Autodesk Inventor part; units mm, degrees
ref_plane "YZ Plane" through (0, 0, 0) normal (1, 0, 0) x (0, 1, 0)
ref_plane "XZ Plane" through (0, 0, 0) normal (0, 1, 0) x (-1, 0, 0)
ref_plane "XY Plane" through (0, 0, 0) normal (0, 0, 1) x (1, 0, 0)
sketch "Sketch1" plane through (0, 0, 0) normal (0, 1, 0) x (-1, 0, 0)
  arc A0 (1.4918, 12.1563) -> (-1.4918, 12.1563) centre (0, 12) ccw
  arc A1 (-1.4918, -12.1563) -> (1.4918, -12.1563) centre (0, -12) ccw
  line L0 (0, -12) -> (0, 12) construction
  line L1 (-2.735, 0.2865) -> (-1.4918, 12.1563)
  line L2 (1.4918, -12.1563) -> (2.735, -0.2865)
  line L3 (-1.4918, -12.1563) -> (-2.735, -0.2865)
  line L4 (2.735, 0.2865) -> (1.4918, 12.1563)
  arc A2 (-2.735, 0.2865) -> (-2.735, -0.2865) centre (0, 0) ccw
  arc A3 (2.735, -0.2865) -> (2.735, 0.2865) centre (0, 0) ccw
  line L5 (2.75, 0) -> (-2.75, 0) construction
  line L6 (-3.0334, -0.3177) -> (-1.7902, -12.1875)
  arc A4 (-1.7902, -12.1875) -> (1.7902, -12.1875) centre (0, -12) ccw
  line L7 (1.7902, -12.1875) -> (3.0334, -0.3177)
  arc A5 (3.0334, -0.3177) -> (3.0334, 0.3177) centre (0, 0) ccw
  line L8 (3.0334, 0.3177) -> (1.7902, 12.1875)
  arc A6 (1.7902, 12.1875) -> (-1.7902, 12.1875) centre (0, 12) ccw
  line L9 (-1.7902, 12.1875) -> (-3.0334, 0.3177)
  arc A7 (-3.0334, 0.3177) -> (-3.0334, -0.3177) centre (0, 0) ccw
  line L10 (-4.25, 27.45) -> (4.25, 27.45)
  line L11 (4.25, 27.45) -> (4.25, 48.45)
  line L12 (4.25, 48.45) -> (-4.25, 48.45)
  line L13 (-4.25, 48.45) -> (-4.25, 27.45)
  line L14 (0, -16.975) -> (0, 53.0999) construction
  line L15 (-7.425, -9.55) -> (-7.425, 45.6749)
  line L16 (7.425, 45.6749) -> (7.425, -9.55)
  arc A8 (-7.425, -9.55) -> (7.425, -9.55) centre (0, -9.55) ccw
  arc A9 (7.425, 45.6749) -> (-7.425, 45.6749) centre (0, 45.6749) ccw
  line L17 (4.45, 48.65) -> (4.45, 27.25)
  line L18 (4.45, 27.25) -> (-4.45, 27.25)
  line L19 (-4.45, 27.25) -> (-4.45, 48.65)
  line L20 (-4.45, 48.65) -> (4.45, 48.65)
  point P0 (0, 0)
  point P1 (0, 27.45)
  point P2 (0, 44.45)
  point P3 (0, 18.0624)
  point P4 (0, -13.8)
  point P5 (0, -16.975)
  dimension "d5" = 3
  dimension "d6" = 3
  dimension "d7" = 24
  dimension "d8" = 5.5
  dimension "d9" = 0.3
  dimension "d10" = 8.5
  dimension "d11" = 21
  dimension "d12" = 4
  dimension "d13" = 44.45
  dimension "d14" = 3.175
  dimension "d15" = 3.175
  dimension "d16" = 0.2
extrude "Extrusion1" add sketch "Sketch1" along normal blind 1.5875 contours L15 A9 L16 A8
sketch "Sketch2" plane through (0, 1.5875, 0) normal (0, 1, 0) x (1, 0, 0)
  line L0 (7.425, -45.6749) -> (7.425, 9.55)
  arc A0 (7.425, 9.55) -> (-7.425, 9.55) centre (0, 9.55) ccw
  line L1 (-7.425, 9.55) -> (-7.425, -45.6749)
  arc A1 (-7.425, -45.6749) -> (7.425, -45.6749) centre (0, -45.6749) ccw
  line L2 (-4.45, -48.65) -> (-4.45, -27.25)
  line L3 (-4.45, -27.25) -> (4.45, -27.25)
  line L4 (4.45, -27.25) -> (4.45, -48.65)
  line L5 (4.45, -48.65) -> (-4.45, -48.65)
  arc A2 (3.0334, -0.3177) -> (3.0334, 0.3177) centre (0, 0) ccw
  line L6 (3.0334, -0.3177) -> (1.7902, -12.1875)
  arc A3 (-1.7902, -12.1875) -> (1.7902, -12.1875) centre (0, -12) ccw
  line L7 (-1.7902, -12.1875) -> (-3.0334, -0.3177)
  arc A4 (-3.0334, 0.3177) -> (-3.0334, -0.3177) centre (0, 0) ccw
  line L8 (-3.0334, 0.3177) -> (-1.7902, 12.1875)
  arc A5 (1.7902, 12.1875) -> (-1.7902, 12.1875) centre (0, 12) ccw
  line L9 (1.7902, 12.1875) -> (3.0334, 0.3177)
extrude "Extrusion2" add sketch "Sketch2" along normal blind 1.5875 contours A1 L1 A0 L0 | L6 A3 L7 A4 L8 A5 L9 A2
properties part number "arm"
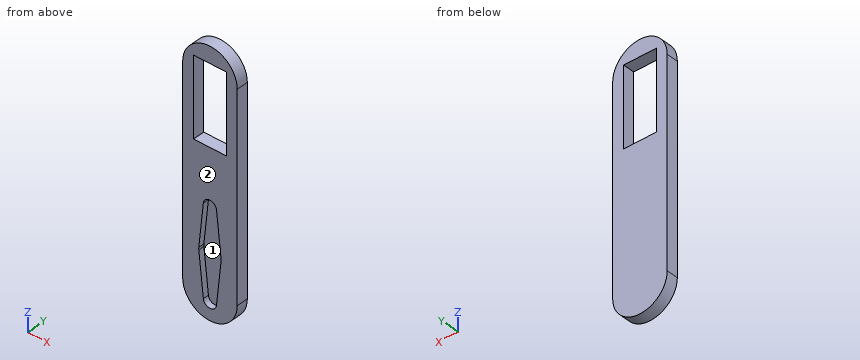
For this review, take the finished solid that the model builds, in its own axes (mm). Face numbers are marked on the shaded views. Give positions to 0.01 mm unless a question says otherwise; leave off trailing zeros. Write each loop counter-clockwise with the first axis right and the second up, starting at its lowest first coordinate (ties: lowest second). Pieces come first, ordered by that corner, then holes. Notation, with made-up numbers: M -28,-22.75 L -6,-22.75 A15 ccw -6,3.25 Z; hole C 65.25,-22.75 d8. An arc over 180 degrees is marked long. Answer as a JSON object with one key per item and string values. Group by question number.
Item 1: Draft analysis for pull direction Z (two halves, no side actions). For the marked faces 1 and 2, state which applies: +Z half, -Z half, draft (parallel to the pull), parting line (faces both ways), or undercut.
Item 2: Consider section D-D on x = 6.75. Write out the cut boundary in (y, z) (3 decimals), plus the area to 3 significant figures.
Item 3: For pin 1 Ø1 at (x, y) = (2, 1) entering from -Z; pin 2 Ø1.5 at (x, y) = (-5, 2.5) entering from +Z; pin 3 Ø1 at (x, y) = (4, 0.5) entering from -Z, all flat-tipped, find the tip position at first contact; note any pin that passes through.
Item 4: For probe 1 along Z at (x, y) = (-0.75, 0.7); probe 2 along Z at (x, y) = (0.5, 1.55); probe 3 along X at (y, z) = (2.5, 37) (3 decimals), list the stretches that pass through material, from the lowest coordinate up. Write a range as [from, to].
Item 5: Consider section C-C on z = -7.5. Write out the cut boundary in (x, y) (1 decimal).
Item 6: Consider section A-A on z = 35. Write out the cut boundary in (x, y) (3 decimals).
Check result:
{
 "1": {"face 1": "undercut", "face 2": "draft"},
 "2": {"outline": "M 0,-12.643 L 3.175,-12.643 L 3.175,48.768 L 0,48.768 Z", "area": "195 mm^2"},
 "3": {"pin 1": "stops at z = -16.82", "pin 2": "stops at z = 51.76", "pin 3": "stops at z = -16.1"},
 "4": {"probe 1": "z = [-16.94, -13.64], [13.64, 27.25], [48.65, 53.06]", "probe 2": "z = [-16.96, -13.73], [13.73, 27.25], [48.65, 53.08]", "probe 3": "x = [-7.425, -4.45], [4.45, 7.425]"},
 "5": {"outline": "M -7.4,0 L -2.3,0 L -2.3,1.6 L 2.3,1.6 L 2.3,0 L 7.4,0 L 7.4,3.2 L -7.4,3.2 Z"},
 "6": {"outline": "M -7.425,0 L -4.45,0 L -4.45,3.175 L -7.425,3.175 Z; M 4.45,0 L 7.425,0 L 7.425,3.175 L 4.45,3.175 Z"}
}
